Source: CAD feature listing. Evaluate the final solid. Frame: model axes, mm. A direction names the side the tool comes from. Round coordinates to 2 decimals unless told otherwise and drop trailing zeros. Write each loop counter-clockwise with the first axis right and the second up, starting at its lowest first coordinate (ties: lowest second). Pieces come first, ordered by that corner, then holes. Notation, with made-up numbers: (-14, 14.25) -> (26, 14.25) arc R29 ccw to (26, 52.25) -> close; hole circle Ø6 at (-39.5, 11). An arc over 180 degrees is marked (long way). Put each result on its own line as item: value.
```python
from build123d import *

# Parameters (mm, degrees)
CROQUIS2_W              = 1
CROQUIS2_H              = 350
SALIENTE_EXTRUIR2_DEPTH = 25
CROQUIS5_R              = 1.5
CORTAR_EXTRUIR2_DEPTH   = 1
CROQUIS1_R              = 1.5
SALIENTE_EXTRUIR3_DEPTH = 1


with BuildPart() as part:
    # Croquis2 → Saliente-Extruir2 (new body)
    with BuildSketch(Plane.XY):
        with Locations((-54.941785307, -113.819624774)):
            Rectangle(CROQUIS2_W, CROQUIS2_H)
    extrude(amount=SALIENTE_EXTRUIR2_DEPTH)

    # Croquis5 → Cortar-Extruir2 (cut)
    with BuildSketch(Plane(origin=(-54.441785307, 0, 0), x_dir=(0, 0, -1), z_dir=(1, 0, 0))):
        with Locations((-20, 43.180375226)):
            Circle(CROQUIS5_R)
        with Locations((-20, -270.819624774)):
            Circle(CROQUIS5_R)
    extrude(amount=-CORTAR_EXTRUIR2_DEPTH, mode=Mode.SUBTRACT)

    # Croquis1 → Saliente-Extruir3 (add)
    with BuildSketch(Plane.XY):
        Polygon((-55.441785307, 61.180375226), (-79.441785307, 37.180375226), (-79.441785307, -264.819624774), (-55.441785307, -288.819624774), align=None)
        with Locations((-74.441785307, 21.180375226)):
            Circle(CROQUIS1_R, mode=Mode.SUBTRACT)
        with Locations((-74.441785307, -248.819624774)):
            Circle(CROQUIS1_R, mode=Mode.SUBTRACT)
        with Locations((-74.441785307, -168.819624774)):
            Circle(CROQUIS1_R, mode=Mode.SUBTRACT)
    extrude(amount=SALIENTE_EXTRUIR3_DEPTH)


solid = part.part
```
Q1. Material intervals for line 1 (Y direction, x = -54.7, z = 20); line 2 (Z direction, x = -56.75, y = -180); line 3 (X direction, y = -261, z = 14.5), sorted ascending. Write a range as [from, to].
Ans:
line 1: y = [-288.82, -272.32], [-269.32, 41.68], [44.68, 61.18]
line 2: z = [0, 1]
line 3: x = [-55.44, -54.44]
Q2. Reachability of faces 1 (the flat face through (-55.442, -116, 13)), 2 (the flat face through (-67.27, 49.35, 0.49)) from +Z, -Z, +X, -X, +Y, -Y: full face, straight path, thin tool, end or side. Return the list, or none.
Ans:
face 1: +Z, -X, +Y, -Y
face 2: +Z, -Z, -X, +Y
Q3. Cut plane C-C on x = -59. Output: boundary loops of the cut face in (y, z).
Ans:
outline: (-285.26, 0) -> (57.62, 0) -> (57.62, 1) -> (-285.26, 1) -> close
Q4. Cut plane A-A on y = -153. Output: boundary loops of the cut face in (x, z), and give its area (3 significant figures).
Ans:
outline: (-79.44, 0) -> (-54.44, 0) -> (-54.44, 25) -> (-55.44, 25) -> (-55.44, 1) -> (-79.44, 1) -> close
area: 49.0 mm^2
Q5. Pin query (flat end, axial travel): pin 1 (4 mm diameter, centred on x = -61, y = -85.5, fed in from -Z); pin 2 (8 mm diameter, centred on x = -60, z = 3.5, fed in from +Y); pin 3 (3 mm diameter, centred on y = -133.5, z = 10.5, fed in from -X); pin 4 (4 mm diameter, centred on x = -66.5, y = -203, fed in from +Z). Return the tip coordinate at first contact, or that it passes through.
Ans:
pin 1: stops at z = 0
pin 2: stops at y = 59.74
pin 3: stops at x = -55.44
pin 4: stops at z = 1
Q6. Cut plane B-B on z = 10.5. Output: boundary loops of the cut face in (x, y).
Ans:
outline: (-55.44, -288.82) -> (-54.44, -288.82) -> (-54.44, 61.18) -> (-55.44, 61.18) -> close
